Part print with two shaded views. Sizes in mm from the minimum x, y, z corner. A direction names the side the tool comes from. Round coordinates to 2 decimals unless told otherwise and drop trailing zeros. Loops run counter-clockwise (first coordinate to the right, second up) from the corner with the lowest first, then second, coordinate; pieces in that order, holes last. Notation, with made-up numbers: (2, 38) -> (39, 38) arc R19 ccw to (39, 62) -> close; hole circle Ø1 at (-22.5, 74). An arc over 180 degrees is marked (long way). Answer as a JSON object with one key per item and string values. Group by question number.
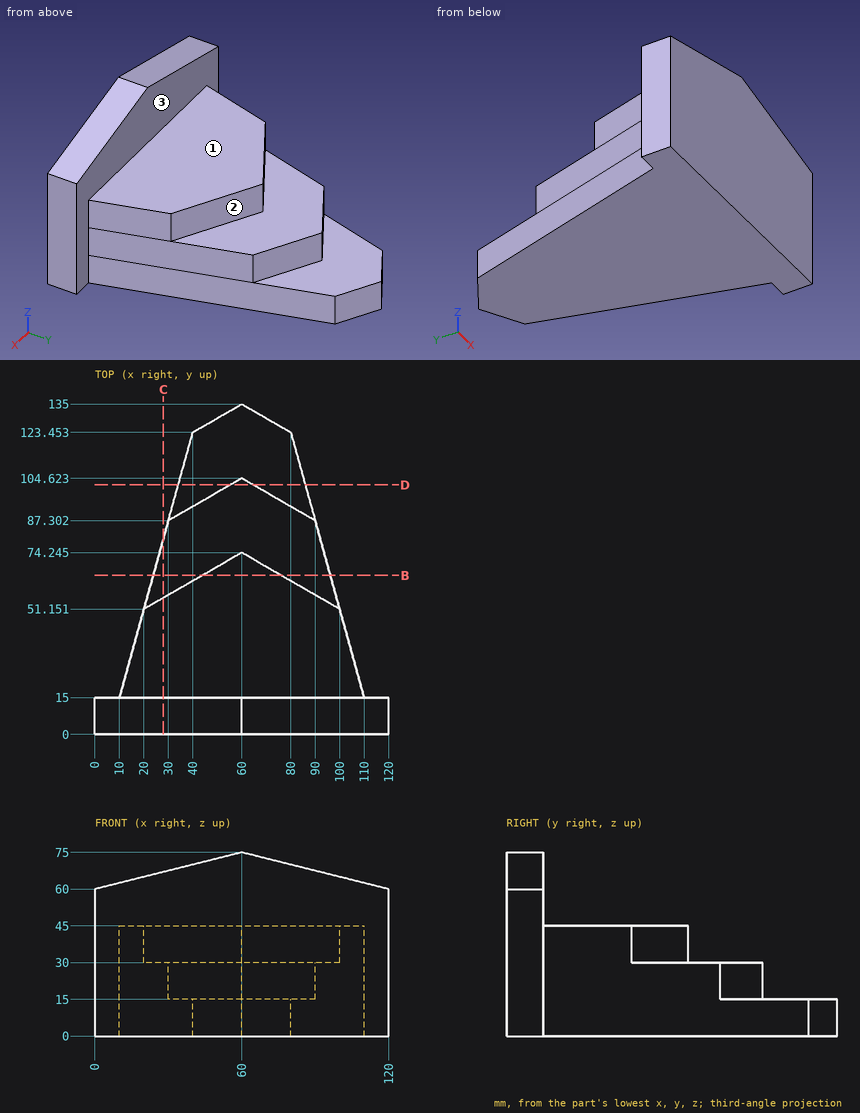
Item 1: Which spindle directions (+Z, -Z, +X, -X, +Y, -Y) get a long thin tool onto all of the face, cutting with end or side? Do the marked faces 1, 2 and 3. Say none if no direction does.
Item 2: Drill centre lines: line 1 (Z direction, x = 23, y = 45.5); line 2 (Y direction, x = 111, z = 23); line 3 (Z direction, x = 87, y = 80.5). Where is each one in solid material? Low to high.
Item 3: Band-saw the part on B-B, the plane y = 65. List the corners of the cut face in (x, z).
Item 4: Drop flat-ended pins along their axis: pin 1 Ø5 at (x, y) = (81.5, 62) entering from +Z; pin 2 Ø6 at (x, z) = (55.5, 42) entering from +Y; pin 3 Ø14.5 at (x, y) = (47, 100.5) entering from +Z. Give the stop position or say it passes through.
Item 5: Band-saw the part on D-D, the plane y = 102. List the corners of the cut face in (x, z) (1 decimal), plus the area to 3 significant figures.
Item 6: Band-saw the part on C-C, the plane x = 28. List the corners of the cut face in (y, z), plus the area to 3 significant figures.
Entries:
{
 "1": {"face 1": "+Z, +X, -X, +Y", "face 2": "+Z, +X, +Y", "face 3": "+Z, +Y"},
 "2": {"line 1": "0 to 45", "line 2": "0 to 15", "line 3": "0 to 30"},
 "3": {"outline": "(23.83, 0) -> (96.17, 0) -> (96.17, 30) -> (76.01, 30) -> (76.01, 45) -> (43.99, 45) -> (43.99, 30) -> (23.83, 30) -> close"},
 "4": {"pin 1": "z = 45", "pin 2": "y = 73.38", "pin 3": "z = 30"},
 "5": {"outline": "(34.1, 0) -> (85.9, 0) -> (85.9, 15) -> (64.5, 15) -> (64.5, 30) -> (55.5, 30) -> (55.5, 15) -> (34.1, 15) -> close", "area": "914 mm²"},
 "6": {"outline": "(0, 0) -> (80.07, 0) -> (80.07, 30) -> (55.77, 30) -> (55.77, 45) -> (15, 45) -> (15, 67) -> (0, 67) -> close", "area": "3,570 mm²"}
}
